Part model, mm, in its own coordinate system. A direction names the side the tool comes from. Give positions to 0.01 mm unless a question says otherwise; leave off trailing zeros. Order: outer loops, then holes, each group sorted by start corner. A loop starts at its lowest first (then second) coordinate and runs counter-clockwise, first axis right, second up. Notation, with made-up numbers: M 23,-26 L 43,-26 A32 cw 43,3 Z; hole C 10.5,58 d4. An arc over 180 degrees is marked long. Answer as a JSON object with one key per item and string values.
from build123d import *

# Parameters (mm, degrees)
SKETCH_1_R        = 3
EXTRUDE_2_DEPTH   = 5
SKETCH_3_R        = 5
EXTRUDE_3_DEPTH   = 2
HOLE_WIZARD_M31_D = 3.4


with BuildPart() as part:
    # Эскиз1 → Бобышка-Вытянуть2 (new body)
    with BuildSketch(Plane.XY):
        with Locations((-15.5, 15.5)):
            Circle(SKETCH_1_R)
    extrude(amount=EXTRUDE_2_DEPTH)

    # Эскиз3 → Бобышка-Вытянуть3 (add)
    with BuildSketch(Plane.XY.offset(-0.053912026)):
        with Locations((-15.5, 15.5)):
            Circle(SKETCH_3_R)
    extrude(amount=EXTRUDE_3_DEPTH)

    # Отверстие с зазором M31 (through all)
    with Locations(Plane(origin=(-3.782161831, -3.025449216, -0.053912026), x_dir=(-0.9755899156330161, 0.2196003563639286, 0), z_dir=(0, 0, -1))):
        with Locations((15.5, 15.5)):
            Hole(HOLE_WIZARD_M31_D / 2)


solid = part.part
1. Cut at D-D on z = 0.4. Give the cut face in (x, y).
Worked answers:
{"outline": "C -15.5,15.5 d10; hole C -15.5,15.5 d3.4"}
2. Cut at B-B on x = -15.5. Give the cut face in (y, z), plus the area to 3 significant figures.
Worked answers:
{"outline": "M 10.5,-0.05 L 13.8,-0.05 L 13.8,5 L 12.5,5 L 12.5,1.95 L 10.5,1.95 Z; M 17.2,-0.05 L 20.5,-0.05 L 20.5,1.95 L 18.5,1.95 L 18.5,5 L 17.2,5 Z", "area": "21.1 mm^2"}
3. Which spindle directions (+Z, -Z, +X, -X, +Y, -Y) get a long thin tool onto all of the face, cutting with end or side? Do faces 4 (the flat face through (-13, 13, 1.946)), 5 (the flat face through (-14, 14, 5)). Say none if no direction does.
Worked answers:
{"face 4": "+Z", "face 5": "+Z, +X, -X, +Y, -Y"}
4. Probe line 1 along Y through (x, z) = (-15.5, 3.1); line 2 along X through (y, z) = (15.5, 3.25); line 3 along Y through (x, z) = (-15.5, 1.65). List the from-to ranges inside material, lowest first.
Worked answers:
{"line 1": "y = 12.5 to 13.8, 17.2 to 18.5", "line 2": "x = -18.5 to -17.2, -13.8 to -12.5", "line 3": "y = 10.5 to 13.8, 17.2 to 20.5"}
5. Cut at A-A on y = 15.5. Give the cut face in (x, z), plus the area to 3 significant figures.
Worked answers:
{"outline": "M -20.5,-0.05 L -17.2,-0.05 L -17.2,5 L -18.5,5 L -18.5,1.95 L -20.5,1.95 Z; M -13.8,-0.05 L -10.5,-0.05 L -10.5,1.95 L -12.5,1.95 L -12.5,5 L -13.8,5 Z", "area": "21.1 mm^2"}
6. Pin check, flat tips, straight feed: P1, Ø3, axis at x = -18, y = 13, coming from the +Z side; P2, Ø1.5, axis at x = -19, y = 13.5, coming from the +Z side; P3, Ø1.5, axis at y = 15, z = 3.5, coming from the +X side; P4, Ø1.5, axis at y = 13.5, z = 1.5, coming from the -X side. Stop position of each tip, or through.
Worked answers:
{"P1": "stops at z = 5", "P2": "stops at z = 1.95", "P3": "stops at x = -12.5", "P4": "stops at x = -20.34"}
7. Two-plate mould, pull along X, no slides. Class faces 1 (the flat face through (-16, 13, -0.054)), 2 (the cylindrical face through (-16.58, 10.62, 0.93)), 3 (the cylindrical face through (-14.294, 16.698, 2.508)): +X half, -X half, draft (parallel to the pull), parting line (faces both ways), or undercut.
Worked answers:
{"face 1": "draft", "face 2": "parting line", "face 3": "undercut"}
8. Cut at C-C on x = -13.5. Give the cut face in (y, z).
Worked answers:
{"outline": "M 10.92,-0.05 L 20.08,-0.05 L 20.08,1.95 L 17.74,1.95 L 17.74,5 L 13.26,5 L 13.26,1.95 L 10.92,1.95 Z"}
